```python
from build123d import *

# Parameters (mm, degrees)
SKETCH2_R               = 47.5
SKETCH2_R_2             = 3.25
BOSS_EXTRUDE1_DEPTH     = 2.5
SKETCH3_R               = 7
CUT_EXTRUDE1_DEPTH      = 5
SKETCH4_R               = 35
BOSS_EXTRUDE2_DEPTH     = 5
SKETCH5_R               = 14
BOSS_EXTRUDE3_DEPTH     = 18
SKETCH6_R               = 7
CUT_EXTRUDE2_DEPTH      = 1
CUT_EXTRUDE2_DEPTH_BACK = 29
FILLET1_R               = 5


with BuildPart() as part:
    # Sketch2 → Boss-Extrude1 (new body, symmetric)
    with BuildSketch(Plane(origin=(0, 0, 0), x_dir=(1, 0, 0), z_dir=(0, 1, 0))):
        Circle(SKETCH2_R)
        with Locations((0, 40)):
            Circle(SKETCH2_R_2, mode=Mode.SUBTRACT)
        with Locations((34.641016151, 20)):
            Circle(SKETCH2_R_2, mode=Mode.SUBTRACT)
        with Locations((34.641016151, -20)):
            Circle(SKETCH2_R_2, mode=Mode.SUBTRACT)
        with Locations((0, -40)):
            Circle(SKETCH2_R_2, mode=Mode.SUBTRACT)
        with Locations((-34.641016151, -20)):
            Circle(SKETCH2_R_2, mode=Mode.SUBTRACT)
        with Locations((-34.641016151, 20)):
            Circle(SKETCH2_R_2, mode=Mode.SUBTRACT)
    extrude(amount=BOSS_EXTRUDE1_DEPTH, both=True)

    # Sketch3 → Cut-Extrude1 (cut)
    with BuildSketch(Plane(origin=(0, 2.5, 0), x_dir=(1, 0, 0), z_dir=(0, 1, 0))):
        Circle(SKETCH3_R)
    extrude(amount=-CUT_EXTRUDE1_DEPTH, mode=Mode.SUBTRACT)

    # Sketch4 → Boss-Extrude2 (add)
    with BuildSketch(Plane(origin=(0, 2.5, 0), x_dir=(1, 0, 0), z_dir=(0, 1, 0))):
        Circle(SKETCH4_R)
    extrude(amount=BOSS_EXTRUDE2_DEPTH)

    # Sketch5 → Boss-Extrude3 (add)
    with BuildSketch(Plane.XZ.offset(2.5)):
        Circle(SKETCH5_R)
    extrude(amount=BOSS_EXTRUDE3_DEPTH)

    # Sketch6 → Cut-Extrude2 (cut, two sides)
    with BuildSketch(Plane.XZ.offset(20.5)) as cut_extrude2_sk:
        Circle(SKETCH6_R)
    extrude(amount=CUT_EXTRUDE2_DEPTH, mode=Mode.SUBTRACT)
    extrude(cut_extrude2_sk.sketch, amount=-CUT_EXTRUDE2_DEPTH_BACK, mode=Mode.SUBTRACT)

    # Fillet1
    fillet1_edges = [part.edges().sort_by_distance(p)[0] for p in [
        (-14, -2.5, 0),
    ]]
    fillet(fillet1_edges, radius=FILLET1_R)


solid = part.part
```
Read the model definition and answer for the solid it produces. Units are mm, in the model's axes. A direction names the side the tool comes from. Give positions to 0.01 mm unless a question says otherwise; leave off trailing zeros. Order: outer loops, then holes, each group sorted by start corner. A loop starts at its lowest first (then second) coordinate and runs counter-clockwise, first axis right, second up.
(1) Find section D-D (x = -36.5). Give the vertices of the cut face in (y, z).
(2) Find section C-C (x = 0). Give the vertices of the cut face in (y, z).
(3) Straight lines are drawn through the part: L1, parallel to X at y = 1.3, z = 20; L2, parallel to Z at x = 0, y = -9; L3, parallel to Y at x = 29.5, z = 36.5. For each, find the intervals that lie inside material, in ascending order.
(4) For a pull along Z with two mould halves and no side action, classify faces 1 (the cylindrical face through (-31.639, -0.035, -18.755)), 2 (the flat face through (-6.4, -20.5, 3.3)), 3 (the cylindrical face through (-10.3, 0.04, 46.37)) as released by +Z, released by -Z, zero draft, split by the parting line, or undercut.
(5) For faces 4 (the cylindrical face through (12.932, -13.909, -5.362)), 5 (the flat face through (20.9, 2.5, -28.4)), 6 (the cylindrical face through (-0.705, -0.035, -36.827)), determine the directions among +Z, -Z, +X, -X, +Y, -Y from which every point of the face is accessible in a straight line to the end or side of a thin tool.
(6) Find section A-A (z = 0). Give the vertices of the cut face in (x, y), plus the area to 3 significant figures.
(7) Given pin 1 (8.5 mm diameter, centred on x = 0, z = 40, fed in from -Y); pin 2 (5 mm diameter, centred on x = 34.64, z = 20, fed in from -Y); pin 3 (2 mm diameter, centred on x = -24, y = 1.5, fed in from +Z); pin 4 (3 mm diameter, centred on x = -28.5, y = -2.5, fed in from -Z), each flat-ended and moving along its own axis, determine where each tip first touches the part or whether it passes through.
(8) Find section B-B (y = 0.25). Give the vertices of the cut face in (x, z).
Result sheet:
1. outline: (-2.5, -30.4) - (2.5, -30.4) - (2.5, -22.67) - (-2.5, -22.67) - close; (-2.5, -17.33) - (2.5, -17.33) - (2.5, 17.33) - (-2.5, 17.33) - close; (-2.5, 22.67) - (2.5, 22.67) - (2.5, 30.4) - (-2.5, 30.4) - close
2. outline: (-20.5, -14) - (-7.5, -14) arc R5 cw to (-2.5, -19) - (-2.5, -36.75) - (2.5, -36.75) - (2.5, -35) - (7.5, -35) - (7.5, -7) - (-20.5, -7) - close; (-20.5, 7) - (7.5, 7) - (7.5, 35) - (2.5, 35) - (2.5, 36.75) - (-2.5, 36.75) - (-2.5, 19) arc R5 cw to (-7.5, 14) - (-20.5, 14) - close; (-2.5, -47.5) - (2.5, -47.5) - (2.5, -43.25) - (-2.5, -43.25) - close; (-2.5, 43.25) - (2.5, 43.25) - (2.5, 47.5) - (-2.5, 47.5) - close
3. L1: x = -43.08 to -37.89, -31.39 to 31.39, 37.89 to 43.08
3. L2: z = -14 to -7, 7 to 14
3. L3: y = -2.5 to 2.5
4. face 1: undercut
4. face 2: zero draft
4. face 3: split by the parting line
5. face 4: -Y
5. face 5: +Y
5. face 6: +Y, -Y
6. outline: (-47.5, -2.5) - (-19, -2.5) arc R5 cw to (-14, -7.5) - (-14, -20.5) - (-7, -20.5) - (-7, 7.5) - (-35, 7.5) - (-35, 2.5) - (-47.5, 2.5) - close; (7, -20.5) - (14, -20.5) - (14, -7.5) arc R5 cw to (19, -2.5) - (47.5, -2.5) - (47.5, 2.5) - (35, 2.5) - (35, 7.5) - (7, 7.5) - close
6. area: 948 mm2
7. pin 1: stops at y = -2.5
7. pin 2: passes through
7. pin 3: stops at z = 41.56
7. pin 4: stops at z = -39.08
8. outline: circle Ø95 at (0, 0); hole circle Ø6.5 at (-34.64, -20); hole circle Ø6.5 at (-34.64, 20); hole circle Ø14 at (0, 0); hole circle Ø6.5 at (0, -40); hole circle Ø6.5 at (0, 40); hole circle Ø6.5 at (34.64, -20); hole circle Ø6.5 at (34.64, 20)
